Model file for the job. Use its own axes, mm. Give positions to 0.01 mm unless a question says otherwise; leave off trailing zeros. Loops run counter-clockwise (first coordinate to the right, second up) from the corner with the lowest first, then second, coordinate; pieces in that order, holes last. Notation, with made-up numbers: M 22,51.5 L 30,51.5 A32 ccw 30,78.5 Z; hole C 56.25,36.25 d11. An arc over 180 degrees is marked long. Answer in a Markdown table with one row per item.
```python
from build123d import *

# Parameters (mm, degrees)
EXTRUDE_1_DEPTH      = 150
EXTRUDE_1_DEPTH_BACK = 50


with BuildPart() as part:
    # 草图1 → 凸台-拉伸1 (new, two sides: drawn at the far end of the back side and taken through both)
    with BuildSketch(Plane(origin=(0, 0, 0), x_dir=(1, 0, 0), z_dir=(0, 1, 0)).offset(-EXTRUDE_1_DEPTH_BACK)):
        Polygon((230.940107676, 0), (115.470053838, 200), (-115.470053838, 200), (-230.940107676, 0), (-115.470053838, -200), (115.470053838, -200), align=None)
    extrude(amount=EXTRUDE_1_DEPTH + EXTRUDE_1_DEPTH_BACK)


solid = part.part
```
Q1. Saw through at C-C (x = -125). Give the cut face in (y, z).
Reported:
| item | result |
|---|---|
| outline | M -50,-183.49 L 150,-183.49 L 150,183.49 L -50,183.49 Z |
Q2. Probe probe 1 along X at (y, z) = (63.5, -32.5); probe 2 along Z at (x, y) = (208, 105); probe 3 along X at (y, z) = (53, 7). List the from-to ranges inside material, lowest first.
Reported:
| item | result |
|---|---|
| probe 1 | -212.18 to 212.18 |
| probe 2 | -39.73 to 39.73 |
| probe 3 | -226.9 to 226.9 |
Q3. Drop flat-ended pins along their axis: pin 1 (10 mm diameter, centred on y = 114.5, z = -35.5, fed in from -X); pin 2 (6 mm diameter, centred on x = 181, y = 37, fed in from +Z); pin 3 (5 mm diameter, centred on x = -126.5, y = 33.5, fed in from +Z). Give the stop position or say it passes through.
Reported:
| item | result |
|---|---|
| pin 1 | x = -213.33 |
| pin 2 | z = 91.69 |
| pin 3 | z = 185.23 |
Q4. Saw through at B-B (z = -141.5). Give the cut face in (x, y), and give its area (3 significant figures).
Reported:
| item | result |
|---|---|
| outline | M -149.25,-50 L 149.25,-50 L 149.25,150 L -149.25,150 Z |
| area | 59,700 mm² |
Q5. Saw through at A-A (y = 106.5). Give the cut face in (x, z).
Reported:
| item | result |
|---|---|
| outline | M -230.94,0 L -115.47,-200 L 115.47,-200 L 230.94,0 L 115.47,200 L -115.47,200 Z |
